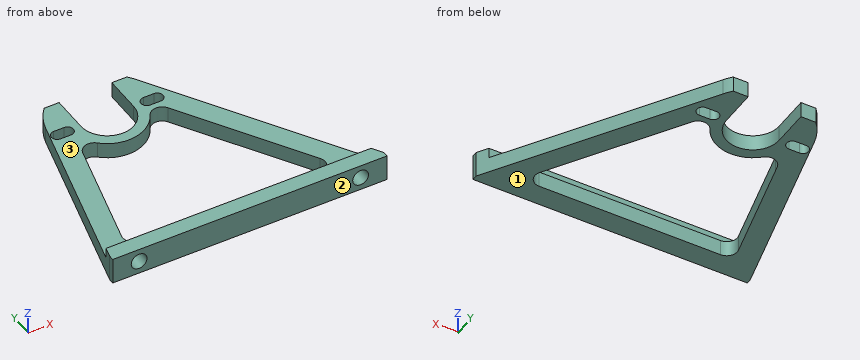
```python
from build123d import *

# Parameters (mm, degrees)
EXTRUDE_1_DEPTH     = 5
SKETCH_2_W          = 105.590665855
SKETCH_2_H          = 53.734325109
CUT_EXTRUDE_1_DEPTH = 2
SKETCH_4_R          = 1.5
CUT_EXTRUDE_2_DEPTH = 3


with BuildPart() as part:
    # 草图1 → 凸台-拉伸1 (new body)
    with BuildSketch(Plane.XY):
        with BuildLine():
            Line((-10.191413347, 2.526874351), (-19, -33))
            Line((-19, -33), (-19, -34))
            Line((-19, -34), (33, -34))
            Line((33, -34), (33, -33))
            Line((33, -33), (8.904718959, 5.563809869))
            ThreePointArc((8.904718959, 5.563809869), (8.396242616, 6.305006736), (7.826237921, 7))
            Line((7.826237921, 7), (5, 7))
            Line((5, 7), (5, 0))
            ThreePointArc((5, 0), (0, -5), (-5, 0))
            Line((-5, 0), (-5, 7))
            Line((-5, 7), (-7.826237921, 7))
            ThreePointArc((-7.826237921, 7), (-9.282303193, 4.908039061), (-10.191413347, 2.526874351))
        make_face()
        with BuildLine():
            Line((-8.452697078, -7.081843943), (-13.519839571, -27.5186906))
            ThreePointArc((-13.519839571, -27.5186906), (-13.153835237, -29.232351654), (-11.578617982, -30))
            Line((-11.578617982, -30), (22.801020138, -30))
            ThreePointArc((22.801020138, -30), (24.55024091, -28.969652872), (24.497157083, -26.940226692))
            Line((24.497157083, -26.940226692), (9.642502803, -3.165776319))
            ThreePointArc((9.642502803, -3.165776319), (7.876643723, -2.22676529), (6.180506778, -3.286538599))
            ThreePointArc((6.180506778, -3.286538599), (1.099422059, -6.91312311), (-4.856029369, -5.041723789))
            ThreePointArc((-4.856029369, -5.041723789), (-6.797250959, -4.560414389), (-8.184687922, -6.0009069))
            Line((-8.184687922, -6.0009069), (-8.452697078, -7.081843943))
        make_face(mode=Mode.SUBTRACT)
        with BuildLine():
            Line((-9.5, 1.1), (-7.5, 1.1))
            ThreePointArc((-7.5, 1.1), (-6.4, 0), (-7.5, -1.1))
            Line((-7.5, -1.1), (-9.5, -1.1))
            ThreePointArc((-9.5, -1.1), (-10.6, 0), (-9.5, 1.1))
        make_face(mode=Mode.SUBTRACT)
        with BuildLine():
            Line((9.5, -1.1), (7.5, -1.1))
            ThreePointArc((7.5, -1.1), (6.4, 0), (7.5, 1.1))
            Line((7.5, 1.1), (9.5, 1.1))
            ThreePointArc((9.5, 1.1), (10.6, 0), (9.5, -1.1))
        make_face(mode=Mode.SUBTRACT)
    extrude(amount=EXTRUDE_1_DEPTH)

    # 草图2 → 切除-拉伸1 (cut)
    with BuildSketch(Plane.XY.offset(5)):
        with Locations((1.500851151, -4.132837446)):
            Rectangle(SKETCH_2_W, SKETCH_2_H)
    extrude(amount=-CUT_EXTRUDE_1_DEPTH, mode=Mode.SUBTRACT)

    # 草图4 → 切除-拉伸2 (cut)
    with BuildSketch(Plane(origin=(0, -34, 0), x_dir=(-1, 0, 0), z_dir=(0, -1, 0))):
        with Locations(Location((14, -2.5, 0), (0, 0, 90))):
            Circle(SKETCH_4_R)
        with Locations(Location((-28, -2.5, 0), (0, 0, 90))):
            Circle(SKETCH_4_R)
    extrude(amount=-CUT_EXTRUDE_2_DEPTH, mode=Mode.SUBTRACT)


solid = part.part
```
Geometry: final body of the model. Coordinates: model frame, mm. Face numbers are marked on the shaded views. Coordinates: 2 decimals unless noted, no trailing zeros. Order: outer loops, then holes, each group sorted by start corner. A loop starts at its lowest first (then second) coordinate and runs counter-clockwise, first axis right, second up. Notation, with made-up numbers: (36, 13) - (66, 13) arc R18 ccw to (66, 38) - close; hole circle Ø8 at (35.25, 14.25). An arc over 180 degrees is marked (long way). Return JSON: item names as keys, results as strings. Group by question number.
1. Material intervals for line 1 along X through (y, z) = (-33.05, 2.5); line 2 along Z through (x, y) = (28, -32); line 3 along X through (y, z) = (-32.5, 2.5), sorted ascending. Write a range as [from, to].
2. Pin query (flat end, axial travel): pin 1 (1.5 mm diameter, centred on y = 5, z = 1, fed in from -X); pin 2 (4 mm diameter, centred on x = 13, y = -12, fed in from +Z); pin 3 (1 mm diameter, centred on x = 5.5, z = 4, fed in from +Y). Return the tip coordinate at first contact, or that it passes through.
3. Cut plane B-B (y = -9). Output: boundary loops of the cut face in (x, z).
4. Pull-direction query (Z, two-part tool) for the marked faces 1, 2 and 3; classes: pulls with the +Z half, pulls with the -Z half, needs draft (parallel to the pull), parting line crosses it, or undercut.
5. Cut plane D-D (z = 1.7). Count the separate pieces of the cut face and the enclosed holes in it, plus the area to 3 significant figures.
6. Cut plane C-C (x = 2). Output: boundary loops of the cut face in (y, z), plus the area to 3 significant figures.
7. Cut plane A-A (x = -3.5). Output: boundary loops of the cut face in (y, z).
Resolved:
{
 "1": {"line 1": "x = [-19, -15.5], [-12.5, 26.5], [29.5, 33]", "line 2": "z = [0, 1], [4, 5]", "line 3": "x = [-18.88, -15.5], [-12.5, 26.5], [29.5, 32.69]"},
 "2": {"pin 1": "stops at x = -9.6", "pin 2": "stops at z = 3", "pin 3": "stops at y = -31"},
 "3": {"outline": "(-13.05, 0) - (-8.93, 0) - (-8.93, 3) - (-13.05, 3) - close; (13.29, 0) - (18, 0) - (18, 3) - (13.29, 3) - close"},
 "4": {"face 1": "pulls with the -Z half", "face 2": "needs draft", "face 3": "pulls with the +Z half"},
 "5": {"separate pieces": "1", "enclosed holes": "3", "area": "557 mm²"},
 "6": {"outline": "(-34, 0) - (-30, 0) - (-30, 3) - (-31, 3) - (-31, 5) - (-34, 5) - close; (-6.71, 0) - (-4.58, 0) - (-4.58, 3) - (-6.71, 3) - close", "area": "24.4 mm²"},
 "7": {"outline": "(-34, 0) - (-30, 0) - (-30, 3) - (-31, 3) - (-31, 5) - (-34, 5) - close; (-6.06, 0) - (-3.57, 0) - (-3.57, 3) - (-6.06, 3) - close"}
}
